from build123d import *

# Parameters (mm, degrees)
SKETCH2_R           = 4
SKETCH2_R_2         = 5.1
BOSS_EXTRUDE3_DEPTH = 5


with BuildPart() as part:
    # Sketch2 → Boss-Extrude3 (new body)
    with BuildSketch(Plane(origin=(0, 0, 0), x_dir=(0, 0, -1), z_dir=(1, 0, 0))):
        Polygon((52, -10), (52, 50), (30, 50), (30, 20), (-10, 20), (-10, -10), align=None)
        with Locations((40, 40)):
            Circle(SKETCH2_R, mode=Mode.SUBTRACT)
        with Locations((40, 20)):
            Circle(SKETCH2_R, mode=Mode.SUBTRACT)
        Circle(SKETCH2_R_2, mode=Mode.SUBTRACT)
    extrude(amount=BOSS_EXTRUDE3_DEPTH)


solid = part.part
For this review, take the finished solid that the model builds, in its own axes (mm). A direction names the side the tool comes from. Round coordinates to 2 decimals unless told otherwise and drop trailing zeros. Order: outer loops, then holes, each group sorted by start corner. A loop starts at its lowest first (then second) coordinate and runs counter-clockwise, first axis right, second up. Notation, with made-up numbers: M 49.5,5.5 L 87.5,5.5 A18 ccw 87.5,22.5 Z; hole C 58,66 d3. An arc over 180 degrees is marked long. Use a Markdown table: item, result. Add a question column.
Item 1: Add section A-A, the plane z = 0. Give the boundary of the cut face in (x, y), then the cut area to 3 significant figures.
Item 2: Add section B-B, the plane y = 0. Give the boundary of the cut face in (x, z), then the cut area to 3 significant figures.
Item 3: Add section D-D, the plane z = -40. Give the boundary of the cut face in (x, y).
Item 4: Mouldability with a two-part tool opening along Y and no side actions: class faces 3 (the cylindrical face through (2.465, 43.966, -39.479)), 4 (the flat face through (2, 5, 10)), 5 (the flat face through (2, 50, -41)) as released by +Y, released by -Y, zero draft, split by the parting line, or undercut.
Item 5: Insertion check: pin 1 (1.5 mm diameter, centred on x = 1.5, z = -18, fed in from +Y); pin 2 (9 mm diameter, centred on y = 0, z = 0, fed in from -X); pin 3 (1.5 mm diameter, centred on x = 1.5, y = 29.5, fed in from +Z). Each pin has a flat end and moves straight along its axis. Give the tip position at first contact, or say it passes through.
Item 6: Add section C-C, the plane x = 3.3. Give the boundary of the cut face in (y, z).
Item 7: To check wall thickness, follow line 1 along Y through (x, z) = (3.8, 0); line 2 along Y through (x, z) = (3.75, -42.5); line 3 along Y through (x, z) = (0.6, 6.5). State the ranges of each line that lie inside material, in increasing order.
Item 8: Tool access review of faces 1 (the flat face through (2, 35, -30)), 2 (the flat face through (2, -10, -21)): name each direction out of +Z, -Z, +X, -X, +Y, -Y from which nothing blocks a thin tool from reaching the whole face with its end or side.
Geometry results:
| question | item | result |
|---|---|---|
| 1 | outline | M 0,-10 L 5,-10 L 5,-5.1 L 0,-5.1 Z; M 0,5.1 L 5,5.1 L 5,20 L 0,20 Z |
| 1 | area | 99.0 mm² |
| 2 | outline | M 0,-52 L 5,-52 L 5,-5.1 L 0,-5.1 Z; M 0,5.1 L 5,5.1 L 5,10 L 0,10 Z |
| 2 | area | 259 mm² |
| 3 | outline | M 0,-10 L 5,-10 L 5,16 L 0,16 Z; M 0,24 L 5,24 L 5,36 L 0,36 Z; M 0,44 L 5,44 L 5,50 L 0,50 Z |
| 4 | face 3 | undercut |
| 4 | face 4 | zero draft |
| 4 | face 5 | released by +Y |
| 5 | pin 1 | stops at y = 20 |
| 5 | pin 2 | passes through |
| 5 | pin 3 | stops at z = -30 |
| 6 | outline | M -10,-52 L 50,-52 L 50,-30 L 20,-30 L 20,10 L -10,10 Z; hole C 0,0 d10.2; hole C 20,-40 d8; hole C 40,-40 d8 |
| 7 | line 1 | y = -10 to -5.1, 5.1 to 20 |
| 7 | line 2 | y = -10 to 16.88, 23.12 to 36.88, 43.12 to 50 |
| 7 | line 3 | y = -10 to 20 |
| 8 | face 1 | +Z, +X, -X, +Y |
| 8 | face 2 | +Z, -Z, +X, -X, -Y |
